Verification items for the finished model (mm, model axes). Give positions to 0.01 mm unless a question says otherwise; leave off trailing zeros. Loops run counter-clockwise (first coordinate to the right, second up) from the corner with the lowest first, then second, coordinate; pieces in that order, holes last. Notation, with made-up numbers: (81, 0) - (90, 0) arc R13 ccw to (90, 18) - close; hole circle Ø3 at (51, 70.25). An arc over 180 degrees is marked (long way). One line per question, with ' | ' between items. Start each with the question number.
1. Section check D-D, the plane z = -375. Enter the section's corners in (x, y).
2. Section check B-B, the plane x = 115. Enter the section's corners in (y, z).
3. Section check C-C, the plane x = 285. Enter the section's corners in (y, z).
4. Thickness scan on line 1 along X through (y, z) = (2.25, -375); line 2 along X through (y, z) = (2, -95); line 3 along Z through (x, y) = (325.5, 1.25). Record the ranges inside material, lowest first. Write a range as from..to.
5. Section check A-A, the plane z = -46. Enter the section's corners in (x, y), then the cut area to 3 significant figures.
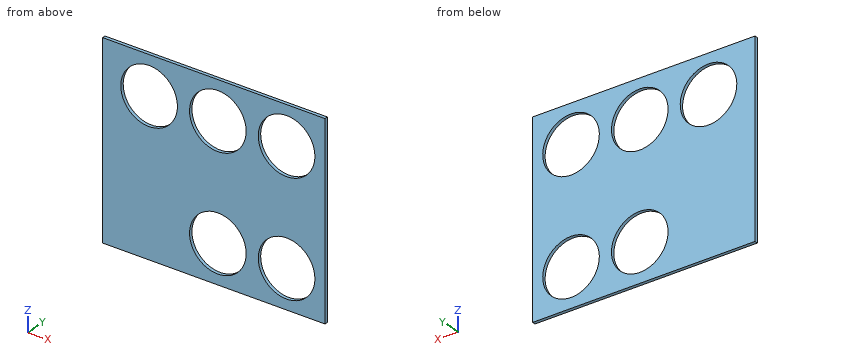
from build123d import *

# Parameters (mm, degrees)
SKETCH1_W           = 550
SKETCH1_H           = 470
BOSS_EXTRUDE1_DEPTH = 8
SKETCH2_R           = 70
CUT_EXTRUDE5_DEPTH  = 8


with BuildPart() as part:
    # Sketch1 → Boss-Extrude1 (new body)
    with BuildSketch(Plane(origin=(0, 0, 0), x_dir=(1, 0, 0), z_dir=(0, 1, 0))):
        with Locations((275, 235)):
            Rectangle(SKETCH1_W, SKETCH1_H)
    extrude(amount=BOSS_EXTRUDE1_DEPTH)

    # Sketch2 → Cut-Extrude5 (cut)
    with BuildSketch(Plane(origin=(0, 0, 0), x_dir=(1, 0, 0), z_dir=(0, 1, 0))):
        with Locations(Location((455, 95, 0), (0, 0, 270))):
            Circle(SKETCH2_R)
        with Locations(Location((285, 95, 0), (0, 0, 270))):
            Circle(SKETCH2_R)
        with Locations(Location((115, 95, 0), (0, 0, 270))):
            Circle(SKETCH2_R)
        with Locations(Location((455, 375, 0), (0, 0, 270))):
            Circle(SKETCH2_R)
        with Locations(Location((285, 375, 0), (0, 0, 270))):
            Circle(SKETCH2_R)
    extrude(amount=CUT_EXTRUDE5_DEPTH, mode=Mode.SUBTRACT)


solid = part.part
Results list:
1) outline: (0, 0) - (215, 0) - (215, 8) - (0, 8) - close; (355, 0) - (385, 0) - (385, 8) - (355, 8) - close; (525, 0) - (550, 0) - (550, 8) - (525, 8) - close
2) outline: (0, -470) - (8, -470) - (8, -165) - (0, -165) - close; (0, -25) - (8, -25) - (8, 0) - (0, 0) - close
3) outline: (0, -470) - (8, -470) - (8, -445) - (0, -445) - close; (0, -305) - (8, -305) - (8, -165) - (0, -165) - close; (0, -25) - (8, -25) - (8, 0) - (0, 0) - close
4) line 1: 0..215, 355..385, 525..550 | line 2: 0..45, 185..215, 355..385, 525..550 | line 3: -470..-432.09, -317.91..-152.09, -37.91..0
5) outline: (0, 0) - (65.01, 0) - (65.01, 8) - (0, 8) - close; (164.99, 0) - (235.01, 0) - (235.01, 8) - (164.99, 8) - close; (334.99, 0) - (405.01, 0) - (405.01, 8) - (334.99, 8) - close; (504.99, 0) - (550, 0) - (550, 8) - (504.99, 8) - close | area: 2,000 mm²
